```python
from build123d import *

# Parameters (mm, degrees)
SKETCH1_R           = 4
BOSS_EXTRUDE1_DEPTH = 12
SKETCH3_R           = 8
BOSS_EXTRUDE2_DEPTH = 7


with BuildPart() as part:
    # Sketch1 → Boss-Extrude1 (new body)
    with BuildSketch(Plane(origin=(0, 0, 0), x_dir=(1, 0, 0), z_dir=(0, 1, 0))):
        Circle(SKETCH1_R)
    extrude(amount=BOSS_EXTRUDE1_DEPTH)

    # Sketch3 → Boss-Extrude2 (add)
    with BuildSketch(Plane(origin=(0, 12, 0), x_dir=(1, 0, 0), z_dir=(0, 1, 0))):
        Circle(SKETCH3_R)
    extrude(amount=BOSS_EXTRUDE2_DEPTH)

    # Sketch4 → Revolve2 (revolve)
    with BuildSketch(Plane.XY):
        with BuildLine():
            Line((0, 28.11938617), (0, 19))
            Line((0, 19), (8, 19))
            ThreePointArc((8, 19), (7.961699903, 28.185937316), (0, 32.767885146))
            Line((0, 32.767885146), (0, 28.11938617))
        make_face()
    revolve(axis=Axis((0, 28.11938617, 0), (0, -1, 0)))


solid = part.part
```
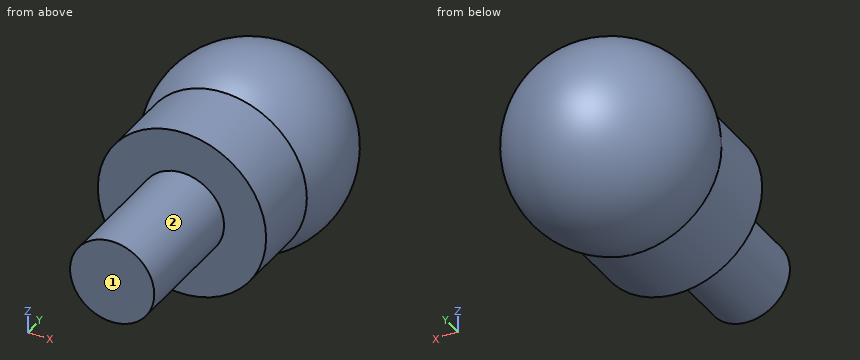
Part model, mm, in its own coordinate system. Face numbers are marked on the shaded views. A direction names the side the tool comes from. Round coordinates to 2 decimals unless told otherwise and drop trailing zeros. Loops run counter-clockwise (first coordinate to the right, second up) from the corner with the lowest first, then second, coordinate; pieces in that order, holes last.
Item 1: Cut at D-D, the plane y = 28. Give the cut face in (x, z).
Item 2: Cut at B-B, the plane x = 0. Give the cut face in (y, z), then the cut area to 3 significant figures.
Item 3: 3-axis set-ups, long thin cutter, end or side, ignore diameter. For the marked faces 1 and 2: which of +Z, -Z, +X, -X, +Y, -Y reach the whole face in a straight line?
Item 4: Cut at A-A, the plane z = 0. Give the cut face in (x, y).
Item 5: Drop flat-ended pins along their axis: P1, Ø1, axis at x = -2, z = -5.5, coming from the -Y side; P2, Ø1, axis at x = 4.5, z = -5.5, coming from the +Y side; P3, Ø4, axis at y = 18.5, z = -1.5, coming from the -X side. Give the stop position or say it passes through.
Item 6: Cut at C-C, the plane y = 16.5. Give the cut face in (x, z), then the cut area to 3 significant figures.
Item 7: Drill centre lines: line 1 (X direction, y = 8, z = 0); line 2 (Y direction, x = -2.25, z = -7); line 3 (Y direction, x = 6.5, z = 5.5). Where is each one in solid material? Low to high.
A:
1. outline: circle Ø16.13 at (0, 0)
2. outline: (0, -4) - (12, -4) - (12, -8) - (19, -8) arc R9.21 ccw (long way) to (19, 8) - (12, 8) - (12, 4) - (0, 4) - close
2. area: 422 mm2
3. face 1: +Z, -Z, +X, -X, -Y
3. face 2: -Y
4. outline: (-8, 12) - (-4, 12) - (-4, 0) - (4, 0) - (4, 12) - (8, 12) - (8, 19) arc R9.21 ccw (long way) to (-8, 19) - close
5. P1: stops at y = 12
5. P2: stops at y = 29.97
5. P3: stops at x = -8.61
6. outline: circle Ø16 at (0, 0)
6. area: 201 mm2
7. line 1: x = -4 to 4
7. line 2: y = 12 to 29.1
7. line 3: y = 20.05 to 27.07
